Can you work these out from the drawing? Everything is in mm from the part's minimum corner. Round coordinates to 2 decimals unless told otherwise and drop trailing zeros. Loops run counter-clockwise (first coordinate to the right, second up) from the corner with the lowest first, then second, coordinate; pieces in that order, holes last. Notation, with made-up numbers: (-4, -20.75) - (13, -20.75) arc R12 cw to (13, -6.75) - close; hole circle Ø9 at (77, 78.5). An arc over 180 degrees is marked (long way). Answer as CSV lines item,"result". Start each with the question number.
1) I'm going to push flat-ended pins straight in: pin 1 Ø1 at (y, z) = (11, 3) entering from -X; pin 2 Ø2 at (x, z) = (11, 3) entering from -Y; pin 3 Ø2 at (y, z) = (14, 1.5) entering from +X. Where does each tip first touch, or does it pass through?
2) Suppose I cut it at D-D, the plane x = 1.25. Write out the boundary of the cut face in (y, z).
3) Suppose I cut it at A-A, the plane x = 9.5. Write out the boundary of the cut face in (y, z), then the cut area to 3 significant figures.
4) We'd pull the mould along Y, two halves only. Please class the marked faces 1, 2 and 3: pulls with the +Y half, pulls with the -Y half, needs draft (parallel to the pull), parting line crosses it, or undercut.
5) Please list where these lines run through material, in increasing order: line 1 along Y through (x, z) = (9.5, 2.7); line 2 along Y through (x, z) = (12.75, 0.9); line 3 along X through (y, z) = (4.75, 0.65).
6) Suppose I cut it at C-C, the plane z = 1. Write out the boundary of the cut face in (x, y), then the cut area to 3 significant figures.
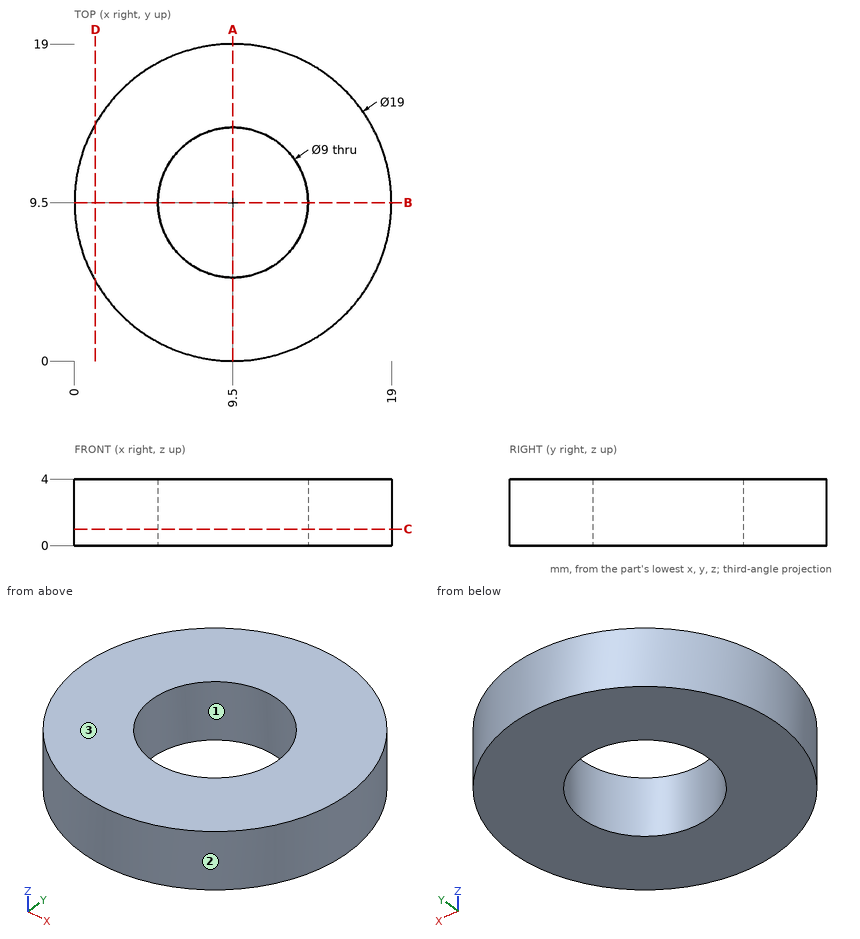
Filled sheet:
1,pin 1,"x = 0.05"
1,pin 2,"y = 0.01"
1,pin 3,"x = 18.33"
2,outline,"(4.79, 0) - (14.21, 0) - (14.21, 4) - (4.79, 4) - close"
3,outline,"(0, 0) - (5, 0) - (5, 4) - (0, 4) - close; (14, 0) - (19, 0) - (19, 4) - (14, 4) - close"
3,area,"40.0 mm²"
4,face 1,"undercut"
4,face 2,"parting line crosses it"
4,face 3,"needs draft"
5,line 1,"0 to 5, 14 to 19"
5,line 2,"0.57 to 6.39, 12.61 to 18.43"
5,line 3,"1.27 to 17.73"
6,outline,"circle Ø19 at (9.5, 9.5); hole circle Ø9 at (9.5, 9.5)"
6,area,"220 mm²"
